```python
from build123d import *

# Parameters (mm, degrees)
PAD006_DEPTH            = 70
POCKET014_DEPTH         = 2.001
SKETCH024_R             = 1.3
POCKET002_DEPTH         = 2.001
SKETCH025_R             = 2.25
POCKET015_DEPTH         = 1
PAD007_DEPTH            = 1.6
LINEARPATTERN_COUNT     = 2
LINEARPATTERN_PITCH     = 68.4
FILLET001_R             = 2
FILLET002_R             = 4
FILLET003_R             = 4
BODY002_PLACEMENT_ANGLE = 180


with BuildPart() as part:
    # Sketch022 → Pad006 (new body)
    with BuildSketch(Plane.YZ):
        with BuildLine():
            ThreePointArc((19, 11.2), (16.217514, 17.917514), (9.5, 20.7))
            Line((-9.5, 20.7), (9.5, 20.7))
            ThreePointArc((-9.5, 20.7), (-16.217514, 17.917514), (-19, 11.2))
            Line((-19, 11.2), (-19, 0))
            Line((-19, 0), (-31, 0))
            Line((-31, 0), (-31, 2))
            Line((-31, 2), (-20.5, 2))
            Line((-20.5, 2), (-20.5, 11.2))
            ThreePointArc((-9.5, 22.2), (-17.278175, 18.978175), (-20.5, 11.2))
            Line((-9.5, 22.2), (9.5, 22.2))
            ThreePointArc((20.5, 11.2), (17.278175, 18.978175), (9.5, 22.2))
            Line((20.5, 2), (20.5, 11.2))
            Line((31, 2), (20.5, 2))
            Line((31, 0), (31, 2))
            Line((19, 0), (31, 0))
            Line((19, 11.2), (19, 0))
        make_face()
    extrude(amount=PAD006_DEPTH)

    # Sketch023 (on Face13 of Pad006) → Pocket014 (cut, through all)
    with BuildSketch(Plane(origin=(0, 0, 2), x_dir=(0, -1, 0), z_dir=(0, 0, 1))):
        Polygon((23, 73), (23, 61.5), (35, 61.5), (35, 49.5), (23, 49.5), (23, 20.5), (35, 20.5), (35, 8.5), (23, 8.5), (23, -3), (46, -3), (46, 73), align=None)
        Polygon((-46, 73), (-23, 73), (-23, 61.5), (-35, 61.5), (-35, 49.5), (-23, 49.5), (-23, 20.5), (-35, 20.5), (-35, 8.5), (-23, 8.5), (-23, -3), (-46, -3), align=None)
    extrude(amount=-POCKET014_DEPTH, mode=Mode.SUBTRACT)

    # Sketch024 (on Face17 of Pocket014) → Pocket002 (cut, through all)
    with BuildSketch(Plane(origin=(0, 0, 2), x_dir=(0, -1, 0), z_dir=(0, 0, 1))):
        with Locations((26, 14)):
            Circle(SKETCH024_R)
        with Locations((-26, 14)):
            Circle(SKETCH024_R)
        with Locations((26, 55.5)):
            Circle(SKETCH024_R)
        with Locations((-26, 55.5)):
            Circle(SKETCH024_R)
    extrude(amount=-POCKET002_DEPTH, mode=Mode.SUBTRACT)

    # Sketch025 (on Face17 of Pocket002) → Pocket015 (cut)
    with BuildSketch(Plane(origin=(0, 0, 2), x_dir=(0, -1, 0), z_dir=(0, 0, 1))):
        with Locations((26, 55.5)):
            Circle(SKETCH025_R)
        with Locations((26, 14)):
            Circle(SKETCH025_R)
        with Locations((-26, 55.5)):
            Circle(SKETCH025_R)
        with Locations((-26, 14)):
            Circle(SKETCH025_R)
    extrude(amount=-POCKET015_DEPTH, mode=Mode.SUBTRACT)

    # Sketch026 → Pad007 (join)
    with BuildSketch(Plane.YZ):
        Polygon((-8.5, 21.7), (8.5, 21.7), (8.5, 19.2), (7, 17.7), (-7, 17.7), (-8.5, 19.2), align=None)
    pad007 = extrude(amount=PAD007_DEPTH)

    # LinearPattern: Pad007 ×2
    with Locations(*[(i * LINEARPATTERN_PITCH, 0, 0) for i in range(1, LINEARPATTERN_COUNT)]):
        add(pad007)

    # Fillet001
    fillet001_edges = [part.edges().sort_by_distance(p)[0] for p in [
        (70, 23, 1),
        (70, -23, 1),
        (0, -23, 1),
        (0, 23, 1),
    ]]
    fillet(fillet001_edges, radius=FILLET001_R)

    # Fillet002
    fillet002_edges = [part.edges().sort_by_distance(p)[0] for p in [
        (8.5, -31, 1),
        (20.5, -31, 1),
        (49.5, -31, 1),
        (61.5, -31, 1),
    ]]
    fillet(fillet002_edges, radius=FILLET002_R)

    # Fillet003
    fillet003_edges = [part.edges().sort_by_distance(p)[0] for p in [
        (61.5, 31, 1),
        (49.5, 31, 1),
        (20.5, 31, 1),
        (8.5, 31, 1),
    ]]
    fillet(fillet003_edges, radius=FILLET003_R)


with BuildPart() as part_1:
    # Body002 placement: moved
    add(part.part.moved(Location((35, 0, -32))).rotate(Axis((35, 0, -32), (0, 1, 0)), BODY002_PLACEMENT_ANGLE))


solid = part_1.part
```
Work out the finished part from the listing and answer in its coordinate system (mm). A direction names the side the tool comes from. Coordinates: 2 decimals unless noted, no trailing zeros. Loops run counter-clockwise (first coordinate to the right, second up) from the corner with the lowest first, then second, coordinate; pieces in that order, holes last. Notation, with made-up numbers: (-37, -10.5) - (-16, -10.5) arc R16 cw to (-16, 9.5) - close; hole circle Ø6 at (76, 46.25). An arc over 180 degrees is marked (long way). Use a Markdown table: item, result.
Item 1: Find section A-A, the plane x = -20.5. State how many separate pieces and enclosed holes the cut face has, and give its area (3 significant figures).
Evaluation:
| item | result |
|---|---|
| separate pieces | 3 |
| enclosed holes | 0 |
| area | 138 mm2 |
Item 2: Find section D-D, the plane x = 12.5. Determine the outline of the cut face in (y, z).
Evaluation:
| item | result |
|---|---|
| outline | (-23, -34) - (-20.5, -34) - (-20.5, -43.2) arc R11 ccw to (-9.5, -54.2) - (9.5, -54.2) arc R11 ccw to (20.5, -43.2) - (20.5, -34) - (23, -34) - (23, -32) - (19, -32) - (19, -43.2) arc R9.5 cw to (9.5, -52.7) - (-9.5, -52.7) arc R9.5 cw to (-19, -43.2) - (-19, -32) - (-23, -32) - close |
Item 3: Find section B-B, the plane z = -38.75. Determine the outline of the cut face in (x, y).
Evaluation:
| item | result |
|---|---|
| outline | (-35, -20.5) - (35, -20.5) - (35, -19) - (-35, -19) - close; (-35, 19) - (35, 19) - (35, 20.5) - (-35, 20.5) - close |
Item 4: For faces 4 (the flat face through (0, -22, -34)), 5 (the flat face through (0, 20.5, -39)), 6 (the flat face through (-19, 26, -33)), 7 (the flat face through (-26.5, 25, -33)), determine the directions among +Z, -Z, +X, -X, +Y, -Y from which every point of the face is accessible in a straight line to the end or side of a thin tool.
Evaluation:
| item | result |
|---|---|
| face 4 | -Z, +X, -X, -Y |
| face 5 | -Z, +X, -X, +Y |
| face 6 | -Z |
| face 7 | +Z, -Z, -X, +Y |
Item 5: The mould has two halves that part along X. Classify faces 1 (the flat face through (-30, -23, -33)), 2 (the cylindrical face through (34.43, 22.4, -32.99)), 3 (the cylindrical face through (21.79, 27.03, -32.51)): +X half, -X half, draft (parallel to the pull), parting line (faces both ways), or undercut.
Evaluation:
| item | result |
|---|---|
| face 1 | draft |
| face 2 | +X half |
| face 3 | undercut |
Item 6: Consider probe 1 along X at (y, z) = (26, -33.65); probe 2 along Y at (x, z) = (-20.5, -32.4); probe 3 along Y at (x, z) = (-1, -41.25). Determine where each line is inside the solid, lowest interval first. Write a range as from..to.
Evaluation:
| item | result |
|---|---|
| probe 1 | x = -26.5..-22.75, -18.25..-14.5, 14.5..18.75, 23.25..26.5 |
| probe 2 | y = -31..-27.3, -24.7..-19, 19..24.7, 27.3..31 |
| probe 3 | y = -20.5..-19, 19..20.5 |
Item 7: Given pin 1 Ø5.5 at (x, z) = (10.5, -36.5) entering from +Y; pin 2 Ø4 at (x, y) = (-20.5, -26) entering from -Z; pin 3 Ø5 at (x, y) = (-20.5, -26.5) entering from -Z, each flat-ended and moving along its own axis, determine where each tip first touches the part or whether it passes through.
Evaluation:
| item | result |
|---|---|
| pin 1 | stops at y = 23 |
| pin 2 | stops at z = -33 |
| pin 3 | stops at z = -34 |
Item 8: Find section C-C, the plane y = 26. Determine the outline of the cut face in (x, z), and give its area (3 significant figures).
Evaluation:
| item | result |
|---|---|
| outline | (-26.5, -34) - (-22.75, -34) - (-22.75, -33) - (-21.8, -33) - (-21.8, -32) - (-26.5, -32) - close; (-19.2, -33) - (-18.25, -33) - (-18.25, -34) - (-14.5, -34) - (-14.5, -32) - (-19.2, -32) - close; (14.5, -34) - (18.75, -34) - (18.75, -33) - (19.7, -33) - (19.7, -32) - (14.5, -32) - close; (22.3, -33) - (23.25, -33) - (23.25, -34) - (26.5, -34) - (26.5, -32) - (22.3, -32) - close |
| area | 33.8 mm2 |
